```python
from build123d import *

# Parameters (mm, degrees)
SKETCH1_R           = 3
BOSS_EXTRUDE1_DEPTH = 3
BOSS_EXTRUDE2_DEPTH = 2
CHAMFER1_SIZE       = 0.5
FILLET1_R           = 1
SKETCH3_R           = 1.6
CUT_EXTRUDE1_DEPTH  = 103.961157725


with BuildPart() as part:
    # Sketch1 → Boss-Extrude1 (new body)
    with BuildSketch(Plane.XY):
        with BuildLine():
            Line((87.658312395, -17.5), (100, -17.5))
            Line((100, -17.5), (100, 17.5))
            Line((100, 17.5), (87.658312395, 17.5))
            ThreePointArc((87.658312395, 17.5), (84.581362835, 17.356617963), (83, 20))
            Line((83, 20), (83, 24))
            Line((83, 24), (-84, 24))
            Line((-84, 24), (-84, -24))
            Line((-84, -24), (83, -24))
            Line((83, -24), (83, -20))
            ThreePointArc((83, -20), (84.581362835, -17.356617963), (87.658312395, -17.5))
        make_face()
        with Locations((-79, -10)):
            Circle(SKETCH1_R, mode=Mode.SUBTRACT)
        with Locations((-79, 10)):
            Circle(SKETCH1_R, mode=Mode.SUBTRACT)
    extrude(amount=BOSS_EXTRUDE1_DEPTH)

    # Sketch2 → Boss-Extrude2 (add)
    with BuildSketch(Plane(origin=(0, 0, 0), x_dir=(-1, 0, 0), z_dir=(0, 0, -1))):
        with BuildLine():
            Line((-73.7, 20), (-73.7, 9.7))
            Line((-73.7, 9.7), (-77.3, 9.7))
            Line((-77.3, 9.7), (-77.3, 15.2))
            Line((-77.3, 15.2), (-97.7, 15.2))
            Line((-97.7, 15.2), (-97.7, -15.2))
            Line((-97.7, -15.2), (-77.3, -15.2))
            Line((-77.3, -15.2), (-77.3, -9.7))
            Line((-77.3, -9.7), (-73.7, -9.7))
            Line((-73.7, -9.7), (-73.7, -20))
            ThreePointArc((-73.7, -20), (-73.494974747, -20.494974747), (-73, -20.7))
            Line((-73, -20.7), (-6, -20.7))
            ThreePointArc((-6, -20.7), (-5.505025253, -20.494974747), (-5.3, -20))
            Line((-5.3, -20), (-5.3, -19))
            ThreePointArc((-5.3, -19), (0, -13.7), (5.3, -19))
            Line((5.3, -19), (5.3, -20))
            ThreePointArc((5.3, -20), (5.505025253, -20.494974747), (6, -20.7))
            Line((6, -20.7), (73, -20.7))
            ThreePointArc((73, -20.7), (73.494974747, -20.494974747), (73.7, -20))
            Line((73.7, -20), (73.7, 20))
            ThreePointArc((73.7, 20), (73.494974747, 20.494974747), (73, 20.7))
            Line((73, 20.7), (6, 20.7))
            ThreePointArc((6, 20.7), (5.505025253, 20.494974747), (5.3, 20))
            Line((5.3, 20), (5.3, 19))
            ThreePointArc((5.3, 19), (0, 13.7), (-5.3, 19))
            Line((-5.3, 19), (-5.3, 20))
            ThreePointArc((-5.3, 20), (-5.505025253, 20.494974747), (-6, 20.7))
            Line((-6, 20.7), (-73, 20.7))
            ThreePointArc((-73, 20.7), (-73.494974747, 20.494974747), (-73.7, 20))
        make_face()
        with BuildLine():
            Line((-7.293833012, 18.7), (-71.7, 18.7))
            Line((-71.7, 18.7), (-71.7, 7.7))
            Line((-71.7, 7.7), (-79.3, 7.7))
            Line((-79.3, 7.7), (-79.3, 13.2))
            Line((-79.3, 13.2), (-95.7, 13.2))
            Line((-95.7, 13.2), (-95.7, -13.2))
            Line((-95.7, -13.2), (-79.3, -13.2))
            Line((-79.3, -13.2), (-79.3, -7.7))
            Line((-79.3, -7.7), (-71.7, -7.7))
            Line((-71.7, -7.7), (-71.7, -18.7))
            Line((-71.7, -18.7), (-7.293833012, -18.7))
            ThreePointArc((-7.293833012, -18.7), (0, -11.7), (7.293833012, -18.7))
            Line((7.293833012, -18.7), (71.7, -18.7))
            Line((71.7, -18.7), (71.7, 18.7))
            Line((71.7, 18.7), (7.293833012, 18.7))
            ThreePointArc((7.293833012, 18.7), (0, 11.7), (-7.293833012, 18.7))
        make_face(mode=Mode.SUBTRACT)
    extrude(amount=BOSS_EXTRUDE2_DEPTH)

    # Chamfer1
    chamfer1_edges = [part.edges().sort_by_distance(p)[0] for p in [
        (73.494974747, 20.494974747, -2),
        (73.7, 14.85, -2),
        (75.5, 9.7, -2),
        (77.3, 12.45, -2),
        (87.5, 15.2, -2),
        (97.7, 0, -2),
        (87.5, -15.2, -2),
        (77.3, -12.45, -2),
        (75.5, -9.7, -2),
        (73.7, -14.85, -2),
        (73.494974747, -20.494974747, -2),
        (39.5, -20.7, -2),
        (5.505025253, -20.494974747, -2),
        (5.3, -19.5, -2),
        (0, -13.7, -2),
        (-5.3, -19.5, -2),
        (-5.505025253, -20.494974747, -2),
        (-39.5, -20.7, -2),
        (-73.494974747, -20.494974747, -2),
        (-73.7, 0, -2),
        (-73.494974747, 20.494974747, -2),
        (-39.5, 20.7, -2),
        (-5.505025253, 20.494974747, -2),
        (-5.3, 19.5, -2),
        (0, 13.7, -2),
        (5.3, 19.5, -2),
        (5.505025253, 20.494974747, -2),
        (39.5, 20.7, -2),
    ]]
    chamfer(chamfer1_edges, length=CHAMFER1_SIZE)

    # Fillet1
    fillet1_edges = [part.edges().sort_by_distance(p)[0] for p in [
        (0, 11.7, 0),
        (39.496916506, 18.7, 0),
        (71.7, 13.2, 0),
        (75.5, 7.7, 0),
        (79.3, 10.45, 0),
        (87.5, 13.2, 0),
        (95.7, 0, 0),
        (87.5, -13.2, 0),
        (79.3, -10.45, 0),
        (75.5, -7.7, 0),
        (71.7, -13.2, 0),
        (39.496916506, -18.7, 0),
        (0, -11.7, 0),
        (-39.496916506, -18.7, 0),
        (-71.7, 0, 0),
        (-39.496916506, 18.7, 0),
    ]]
    fillet(fillet1_edges, radius=FILLET1_R)

    # Sketch3 → Cut-Extrude1 (cut, through all)
    with BuildSketch(Plane.XY.offset(3)):
        with Locations((-79, 19)):
            Circle(SKETCH3_R)
        with Locations((-79, -19)):
            Circle(SKETCH3_R)
        with Locations((79, 19)):
            Circle(SKETCH3_R)
        with Locations((79, -19)):
            Circle(SKETCH3_R)
        with Locations((0, 19)):
            Circle(SKETCH3_R)
        with Locations((0, -19)):
            Circle(SKETCH3_R)
    extrude(amount=-CUT_EXTRUDE1_DEPTH, mode=Mode.SUBTRACT)


solid = part.part
```
Read the model definition and answer for the solid it produces. Units are mm, in the model's axes. A direction names the side the tool comes from. Round coordinates to 2 decimals unless told otherwise and drop trailing zeros. Write each loop counter-clockwise with the first axis right and the second up, starting at its lowest first coordinate (ties: lowest second). Pieces come first, ordered by that corner, then holes. Notation, with made-up numbers: (49, 87.5) - (97, 87.5) arc R20 cw to (97, 99.5) - close; hole circle Ø6 at (67, 43). An arc over 180 degrees is marked (long way). One line per item, written item: value.
Q1. For a pull along X with two mould halves and no side action, classify faces 1 (the flat face through (83, 22, 1)), 2 (the cylindrical face through (-82, -10, 1)), 3 (the flat face through (0, 12, -2)) as pulls with the +X half, pulls with the -X half, needs draft (parallel to the pull), parting line crosses it, or undercut.
The answers:
face 1: pulls with the +X half
face 2: undercut
face 3: needs draft
Q2. Find section A-A (z = 1.3). Count the separate pieces of the cut face and the enclosed holes in it, and give its area (3 significant figures).
The answers:
separate pieces: 1
enclosed holes: 8
area: 8,510 mm2
Q3. Find section B-B (x = -79). Determine the outline of the cut face in (y, z).
The answers:
outline: (-24, 0) - (-20.6, 0) - (-20.6, 3) - (-24, 3) - close; (-17.4, 0) - (-13, 0) - (-13, 3) - (-17.4, 3) - close; (-7, 0) - (7, 0) - (7, 3) - (-7, 3) - close; (13, 0) - (17.4, 0) - (17.4, 3) - (13, 3) - close; (20.6, 0) - (24, 0) - (24, 3) - (20.6, 3) - close
Q4. Find section D-D (x = 0). Determine the outline of the cut face in (y, z).
The answers:
outline: (-24, 0) - (-20.6, 0) - (-20.6, 3) - (-24, 3) - close; (-17.4, 0) - (-13.7, 0) - (-13.7, -1.5) - (-13.2, -2) - (-11.7, -2) - (-11.7, -1) arc R1 cw to (-10.7, 0) - (10.7, 0) arc R1 cw to (11.7, -1) - (11.7, -2) - (13.2, -2) - (13.7, -1.5) - (13.7, 0) - (17.4, 0) - (17.4, 3) - (-17.4, 3) - close; (20.6, 0) - (24, 0) - (24, 3) - (20.6, 3) - close
Q5. Which of the six approach directions +Z, -Z, +X, -X, +Y, -Y give full straight-line access (tool end or side, diameter ignored) to faces 4 (the cylindrical face through (0.16, -11.7, -1.49)), 5 (the cylindrical face through (80.526, 19.481, 1.521)), 6 (the cylindrical face through (-0.1, 13.7, -0.7)), 7 (the flat face through (83, -22, 1))?
The answers:
face 4: -Z
face 5: +Z, -Z
face 6: -Z, +Y
face 7: +Z, -Z, +X, -Y
Q6. Straight lines are drawn through the part: line 1 (Y direction, x = 0, z = 1.85); line 2 (X direction, y = -19, z = -0.7); line 3 (Z direction, x = 81.5, y = -11.5). For each, find the intervals that lie inside material, in ascending order. Write a range as from..to.
The answers:
line 1: y = -24..-20.6, -17.4..17.4, 20.6..24
line 2: x = -73.7..-5.3, 5.3..73.7
line 3: z = 0..3
Q7. Each of these flat-tipped pins is pushed along its axis until it touches: P1, Ø4, axis at x = 79, y = 19, coming from the +Z side; P2, Ø0.8, axis at x = 75, z = -0.5, coming from the +Y side; P3, Ø0.8, axis at x = -44, z = -0.5, coming from the +Y side; P4, Ø0.9, axis at x = 91.5, z = 1.5, coming from the -Y side. Where does it stop, or does it pass through?
The answers:
P1: stops at z = 3
P2: stops at y = 9.7
P3: stops at y = 20.7
P4: stops at y = -17.5
Q8. Find section C-C (x = 19.5). Determine the outline of the cut face in (y, z), and give its area (3 significant figures).
The answers:
outline: (-24, 0) - (-20.7, 0) - (-20.7, -1.5) - (-20.2, -2) - (-18.7, -2) - (-18.7, -1) arc R1 cw to (-17.7, 0) - (17.7, 0) arc R1 cw to (18.7, -1) - (18.7, -2) - (20.2, -2) - (20.7, -1.5) - (20.7, 0) - (24, 0) - (24, 3) - (-24, 3) - close
area: 152 mm2
